For this review, take the finished solid that the model builds, in its own axes (mm). Face numbers are marked on the shaded views. A direction names the side the tool comes from. Round coordinates to 2 decimals unless told otherwise and drop trailing zeros. Loops run counter-clockwise (first coordinate to the right, second up) from the corner with the lowest first, then second, coordinate; pieces in that order, holes last.
1) Insertion check: pin 1 (5 mm diameter, centred on y = -7, z = 21, fed in from -X); pin 2 (6.5 mm diameter, centred on y = 4.5, z = 5.5, fed in from -X); pin 3 (12 mm diameter, centred on x = -11.5, y = 23, fed in from +Z). Each pin has a flat end and moves straight along its axis. Give the tip position at first contact, or say it passes through.
2) Take a section at D-D (x = -44). State the section outline as (y, z) points, then the cut area to 3 significant figures.
3) Wall thickness on L1, parallel to Y at x = -36, z = 15.5; L2, parallel to Z at x = -22, y = 5; L3, parallel to X at y = 34, z = -1.5: over which ranges is each line inside the solid? List them lowest first.
4) Take a section at A-A (z = -7.5). State the section outline as (x, y) points.
5) Take a section at C-C (y = -10). State the section outline as (x, z) points.
6) Mouldability with a two-part tool opening along X and no side actions: class the marked faces 6, 7 and 8 as pulls with the +X half, pulls with the -X half, needs draft (parallel to the pull), parting line crosses it, or undercut.
7) Take a section at B-B (x = 21). State the section outline as (y, z) points, then the cut area to 3 significant figures.
8) Tool access review of the marked faces 1, 2, 3, 4 and 5: name each direction out of +Z, -Z, +X, -X, +Y, -Y from which nothing blocks a thin tool from reaching the whole face with its end or side.
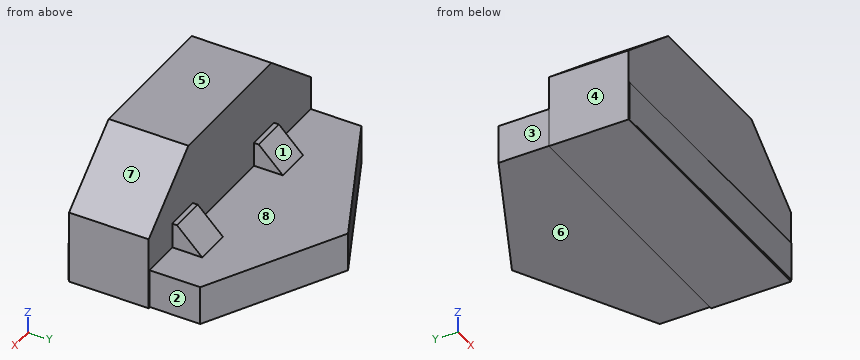
```python
from build123d import *

# Parameters (mm, degrees)
F1_DEPTH    = 25.4
F3_DEPTH    = 12.446
F4_W        = 11.3675398752
F4_H        = 8.0155739561
F4_W_2      = 11.0760703683
F4_H_2      = 7.7240983956
F5_DEPTH    = 14.224
F6_T4_DEPTH = 76.6882877695
F7_T4_DEPTH = 76.3968182626


# Not quite as in the source:
# - a fillet or chamfer that OpenCascade refuses, or shapes differently, is made with other operations: its cross-section is extruded or revolved along the edge and cut away or added


with BuildPart() as f1:
    # F0 (on Front) → F1 (new body)
    with BuildSketch(Plane.XZ):
        Polygon((-56.9788375091, 10.6936474436), (-56.9788375091, -12.6478849719), (32.2034358534, -12.6478849719), (32.2034358534, 10.6936474436), (10.4033187203, 28.9705070476), (-35.1787281407, 28.9705070476), align=None)
    extrude(amount=F1_DEPTH)

    # F2 (on Top) → F3 (join)
    with BuildSketch(Plane.XY):
        Polygon((-56.8377040327, 0), (-56.8377040327, -25.5040973425), (31.7708179355, -25.7955752313), (31.7708179355, 0), align=None)
        Polygon((-56.8377040327, 16.1768849939), (-56.8377040327, 0), (31.7708179355, 0), (31.7708179355, 16.1768849939), (-10.7845906168, 38.6204943061), align=None)
    extrude(amount=-F3_DEPTH)

    # F4 (on Front) → F5 (join)
    with BuildSketch(Plane.XZ):
        with Locations((13.5536068119, 4.007786978)):
            Rectangle(F4_W, F4_H)
        with Locations((-31.1878696084, 3.8620491978)):
            Rectangle(F4_W_2, F4_H_2)
    extrude(amount=-F5_DEPTH)

    # F6: chamfer of 12.7 on 1 edges, made by hand


with BuildPart() as f6_tool2:
    # F6_s3 → F6_t4 (new body)
    with BuildSketch(Plane.YZ.offset(51.8977506967)):
        Polygon((1.524, 8.0155739561), (14.224, -4.6844260439), (14.224, 8.0155739561), align=None)
    extrude(amount=-F6_T4_DEPTH)

    split(bisect_by=Plane.XY, keep=Keep.TOP)


with BuildPart() as f1_1:
    add(f1.part)

    # F6_t1: cut F6_tool2
    add(f6_tool2.part, mode=Mode.SUBTRACT)

    # F7: chamfer of 12.7 on 1 edges, made by hand


with BuildPart() as f7_tool2:
    # F7_s3 → F7_t4 (new body)
    with BuildSketch(Plane.YZ.offset(7.0105395229)):
        Polygon((14.224, -4.9759016044), (1.524, 7.7240983956), (14.224, 7.7240983956), align=None)
    extrude(amount=-F7_T4_DEPTH)

    split(bisect_by=Plane.XY, keep=Keep.TOP)


with BuildPart() as f1_2:
    add(f1_1.part)

    # F7_t1: cut F7_tool2
    add(f7_tool2.part, mode=Mode.SUBTRACT)


solid = f1_2.part
```
Response:
1. pin 1: stops at x = -47.67
1. pin 2: stops at x = -36.73
1. pin 3: stops at z = 0
2. outline: (-25.55, -12.45) - (-25.4, -12.45) - (-25.4, -12.65) - (0, -12.65) - (0, -12.45) - (22.43, -12.45) - (22.43, 0) - (0, 0) - (0, 21.57) - (-25.4, 21.57) - (-25.4, 0) - (-25.55, 0) - close
2. area: 1,150 mm2
3. L1: y = -25.4 to 0
3. L2: z = -12.45 to 0
3. L3: x = -20.27 to -2.02
4. outline: (-56.98, -25.4) - (-56.84, -25.4) - (-56.84, -25.5) - (31.77, -25.8) - (31.77, -25.4) - (32.2, -25.4) - (32.2, 0) - (31.77, 0) - (31.77, 16.18) - (-10.78, 38.62) - (-56.84, 16.18) - (-56.84, 0) - (-56.98, 0) - close
5. outline: (-56.98, -12.65) - (32.2, -12.65) - (32.2, 10.69) - (10.4, 28.97) - (-35.18, 28.97) - (-56.98, 10.69) - close
6. face 6: needs draft
6. face 7: pulls with the +X half
6. face 8: undercut
7. outline: (-25.76, -12.45) - (-25.4, -12.45) - (-25.4, -12.65) - (0, -12.65) - (0, -12.45) - (21.86, -12.45) - (21.86, 0) - (0, 0) - (0, 20.09) - (-25.4, 20.09) - (-25.4, 0) - (-25.76, 0) - close
7. area: 1,110 mm2
8. face 1: +Z, -X, +Y
8. face 2: +Z, -Z, +X, +Y
8. face 3: +Z, -Z, -X, +Y
8. face 4: +Z, -Z, -X, +Y, -Y
8. face 5: +Z, +X, -X, +Y, -Y
